For this review, take the finished solid that the model builds, in its own axes (mm). Face numbers are marked on the shaded views. A direction names the side the tool comes from. Coordinates: 2 decimals unless noted, no trailing zeros. Write each loop counter-clockwise with the first axis right and the second up, starting at its lowest first coordinate (ties: lowest second). Pieces come first, ordered by that corner, then holes. Notation, with made-up numbers: M 25.25,63 L 43.25,63 A31 ccw 43.25,97 Z; hole C 76.25,-17.5 d3. An arc over 180 degrees is marked long. Return JSON: item names as keys, results as strings.
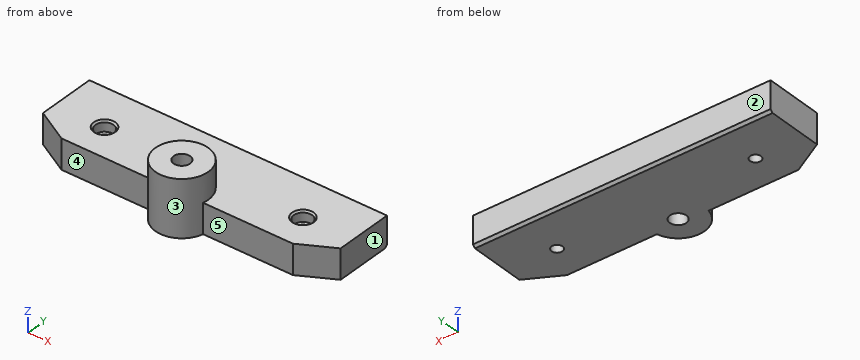
```python
from build123d import *

# Parameters (mm, degrees)
SKETCH1_W                                    = 180
SKETCH1_H                                    = 46
BOSS_EXTRUDE1_DEPTH                          = 18
CUT_EXTRUDE1_DEPTH                           = 95.620293806
CUT_EXTRUDE1_DEPTH_BACK                      = 18
CUT_EXTRUDE2_DEPTH                           = 95.620293806
CUT_EXTRUDE2_DEPTH_BACK                      = 18
SKETCH4_R                                    = 16
BOSS_EXTRUDE2_DEPTH                          = 18
BOSS_EXTRUDE3_START                          = 16
SKETCH5_R                                    = 16
BOSS_EXTRUDE3_DEPTH                          = 16
SKETCH6_R                                    = 5
CUT_EXTRUDE3_DEPTH                           = 103.548768886
CBORE_FOR_M6_HEX_SOCKET_HEAD_CAP_SCR_2_COUNT = 2
CBORE_FOR_M6_HEX_SOCKET_HEAD_CAP_SCR_2_PITCH = 120
CHAMFER1_SIZE                                = 1.5


with BuildPart() as part:
    # Sketch1 → Boss-Extrude1 (new body)
    with BuildSketch(Plane.XY):
        Rectangle(SKETCH1_W, SKETCH1_H)
    extrude(amount=BOSS_EXTRUDE1_DEPTH)

    # Sketch2 → Cut-Extrude1 (cut, two sides: drawn at the far end of the back side and taken through both)
    with BuildSketch(Plane.XY.offset(18).offset(-CUT_EXTRUDE1_DEPTH_BACK)):
        Polygon((-420.107698739, 169.559234306), (-90, -12), (-70, -23), (260.107698739, -204.559234306), (-103.010769874, -864.774631783), (-783.226167351, -490.656163171), align=None)
    extrude(amount=CUT_EXTRUDE1_DEPTH + CUT_EXTRUDE1_DEPTH_BACK, mode=Mode.SUBTRACT)

    # Sketch3 → Cut-Extrude2 (cut, two sides: drawn at the far end of the back side and taken through both)
    with BuildSketch(Plane.XY.offset(18).offset(-CUT_EXTRUDE2_DEPTH_BACK)):
        Polygon((420.107698739, 169.559234306), (90, -12), (70, -23), (-260.107698739, -204.559234306), (103.010769874, -864.774631783), (783.226167351, -490.656163171), align=None)
    extrude(amount=CUT_EXTRUDE2_DEPTH + CUT_EXTRUDE2_DEPTH_BACK, mode=Mode.SUBTRACT)

    # Sketch4 → Boss-Extrude2 (add)
    with BuildSketch(Plane.XY.offset(18)):
        with Locations((0, -19.5)):
            Circle(SKETCH4_R)
    extrude(amount=-BOSS_EXTRUDE2_DEPTH)

    # Sketch5 → Boss-Extrude3 (add)
    with BuildSketch(Plane.XY.offset(18).offset(BOSS_EXTRUDE3_START)):
        with Locations((0, -19.5)):
            Circle(SKETCH5_R)
    extrude(amount=-BOSS_EXTRUDE3_DEPTH)

    # Sketch6 → Cut-Extrude3 (cut, through all)
    with BuildSketch(Plane.XY.offset(34)):
        with Locations((0, -19.5)):
            Circle(SKETCH6_R)
    extrude(amount=-CUT_EXTRUDE3_DEPTH, mode=Mode.SUBTRACT)

    # Sketch8 → CBORE for M6 Hex Socket Head Cap Screw1 (revolve, cut)
    with BuildSketch(Plane(origin=(-60, -3, 18), x_dir=(0, -1, 0), z_dir=(1, 0, 0))):
        Polygon((0, 0), (0, 18), (3.3, 18), (3.3, 6.4), (5.5, 6.4), (5.5, 1.025), (6.525, 0), align=None)
    cbore_for_m6_hex_socket_head_cap_screw1 = revolve(axis=Axis((-60, -3, 24.35), (0, 0, -1)), mode=Mode.SUBTRACT)

    # CBORE for M6 Hex Socket Head Cap Scr 2: CBORE for M6 Hex Socket Head Cap Screw1 ×2
    with Locations(*[(i * CBORE_FOR_M6_HEX_SOCKET_HEAD_CAP_SCR_2_PITCH, 0, 0) for i in range(1, CBORE_FOR_M6_HEX_SOCKET_HEAD_CAP_SCR_2_COUNT)]):
        add(cbore_for_m6_hex_socket_head_cap_screw1, mode=Mode.SUBTRACT)

    # Chamfer1
    chamfer1_edges = [part.edges().sort_by_distance(p)[0] for p in [
        (0, 23, 0),
    ]]
    chamfer(chamfer1_edges, length=CHAMFER1_SIZE)


solid = part.part
```
1. Clearance check with flat-ended pins moving along their axes: pin 1 Ø9 at (x, y) = (60, -3) entering from +Z; pin 2 Ø12 at (y, z) = (-15.5, 25.5) entering from -X; pin 3 Ø2 at (y, z) = (-25.5, 17.5) entering from -X; pin 4 Ø8 at (x, y) = (0, -19.5) entering from +Z. State where each tip first meets the part, or that it passes through.
Checks:
{"pin 1": "z = 11.6", "pin 2": "x = -16", "pin 3": "x = -15.2", "pin 4": "through"}
2. We need section C-C (y = -19.5). State the section outline as (x, z) points, plus the area to 3 significant figures.
Checks:
{"outline": "M -76.36,0 L -5,0 L -5,34 L -16,34 L -16,18 L -76.36,18 Z; M 5,0 L 76.36,0 L 76.36,18 L 16,18 L 16,34 L 5,34 Z", "area": "2,920 mm2"}
3. We need section A-A (z = 7). State the section outline as (x, y) points.
Checks:
{"outline": "M -90,-12 L -70,-23 L -15.61,-23 A16 ccw 15.61,-23 L 70,-23 L 90,-12 L 90,23 L -90,23 Z; hole C -60,-3 d6.6; hole C 0,-19.5 d10; hole C 60,-3 d6.6"}
4. For the marked faces 1, 2, 3, 4 and 5, list the 3-axis set-ups (+Z, -Z, +X, -X, +Y, -Y) from which the entire face can be reached by the end or side of a thin tool; tool diameter is ignored.
Checks:
{"face 1": "+Z, -Z, +X, +Y, -Y", "face 2": "+Z, -Z, +X, -X, +Y", "face 3": "+Z", "face 4": "+Z, -Z, -X, -Y", "face 5": "+Z, -Z, +X, -Y"}
5. Wall thickness on L1, parallel to X at y = -3, z = 13.1; L2, parallel to X at y = -3, z = 5; L3, parallel to Y at x = 60, z = 14: over which ranges is each line inside the solid? List them lowest first. Write a range as from..to.
Checks:
{"L1": "-90..-65.5, -54.5..54.5, 65.5..90", "L2": "-90..-63.3, -56.7..56.7, 63.3..90", "L3": "-23..-8.5, 2.5..23"}
6. We need section B-B (x = 60). State the section outline as (y, z) points (3 decimals).
Checks:
{"outline": "M -23,0 L -6.3,0 L -6.3,11.6 L -8.5,11.6 L -8.5,16.975 L -9.525,18 L -23,18 Z; M 0.3,0 L 21.5,0 L 23,1.5 L 23,18 L 3.525,18 L 2.5,16.975 L 2.5,11.6 L 0.3,11.6 Z"}
7. We need section D-D (z = 26). State the section outline as (x, y) points, plus the area to 3 significant figures.
Checks:
{"outline": "C 0,-19.5 d32; hole C 0,-19.5 d10", "area": "726 mm2"}
